Design review of the part shown in the three views and the two pictorial views. Dimensions are in mm from the part's minimum x, y and z. Give positions to 0.01 mm unless a question says otherwise; leave off trailing zeros. Order: outer loops, then holes, each group sorted by start corner. A loop starts at its lowest first (then second) coordinate and runs counter-clockwise, first axis right, second up.
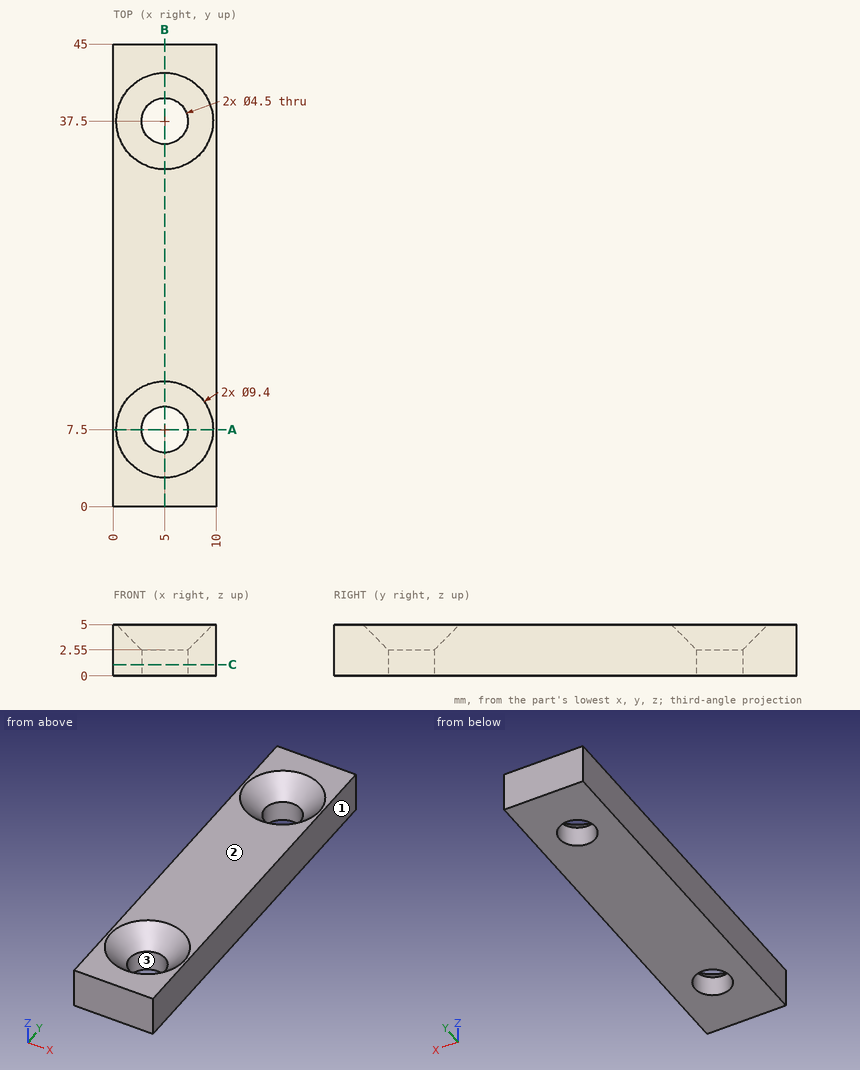
Item 1: Draft analysis for pull direction X (two halves, no side actions). For the marked faces 1, 2 and 3, state which applies: released by +X, released by -X, zero draft, split by the parting line, or undercut.
Values found:
face 1: released by +X
face 2: zero draft
face 3: undercut
Item 2: Take a section at A-A (y = 7.5). Give the boundary of the cut face in (x, z).
Values found:
outline: (0, 0) - (2.75, 0) - (2.75, 2.55) - (0.3, 5) - (0, 5) - close; (7.25, 0) - (10, 0) - (10, 5) - (9.7, 5) - (7.25, 2.55) - close
Item 3: Take a section at C-C (z = 1.1). Give the boundary of the cut face in (x, y).
Values found:
outline: (0, 0) - (10, 0) - (10, 45) - (0, 45) - close; hole circle Ø4.5 at (5, 7.5); hole circle Ø4.5 at (5, 37.5)
Item 4: Clearance check with flat-ended pins moving along their axes: pin 1 Ø5 at (x, y) = (5, 7.5) entering from +Z; pin 2 Ø5 at (x, y) = (5, 37.5) entering from -Z. State where each tip first meets the part, or that it passes through.
Values found:
pin 1: stops at z = 2.8
pin 2: stops at z = 0
Item 5: Take a section at B-B (x = 5). Give the boundary of the cut face in (y, z).
Values found:
outline: (0, 0) - (5.25, 0) - (5.25, 2.55) - (2.8, 5) - (0, 5) - close; (9.75, 0) - (35.25, 0) - (35.25, 2.55) - (32.8, 5) - (12.2, 5) - (9.75, 2.55) - close; (39.75, 0) - (45, 0) - (45, 5) - (42.2, 5) - (39.75, 2.55) - close
Item 6: For line 1 (Y direction, x = 5, z = 1.25); line 2 (X direction, y = 37.5, z = 0.65); line 3 (Y direction, x = 4.75, z = 3.25), list the stretches that pass through material, from the lowest coordinate up.
Values found:
line 1: y = 0 to 5.25, 9.75 to 35.25, 39.75 to 45
line 2: x = 0 to 2.75, 7.25 to 10
line 3: y = 0 to 4.56, 10.44 to 34.56, 40.44 to 45
